```python
from build123d import *

# Parameters (mm, degrees)
SKETCH1_W           = 55.5
SKETCH1_H           = 25.6
SKETCH1_R           = 10
SKETCH1_W_2         = 5
SKETCH1_H_2         = 20
BOSS_EXTRUDE1_DEPTH = 21.5
BOSS_EXTRUDE2_START = 3
SKETCH1_2_W         = 5
SKETCH1_2_H         = 20
SKETCH1_2_R         = 10
BOSS_EXTRUDE2_DEPTH = 18.5


with BuildPart() as part:
    # Sketch1 → Boss-Extrude1 (new body)
    with BuildSketch(Plane.XY):
        Rectangle(SKETCH1_W, SKETCH1_H)
        with Locations((15.75, 0)):
            Circle(SKETCH1_R, mode=Mode.SUBTRACT)
        with Locations((-22.25, 0)):
            Rectangle(SKETCH1_W_2, SKETCH1_H_2, mode=Mode.SUBTRACT)
    extrude(amount=BOSS_EXTRUDE1_DEPTH)

    # Sketch1<2> → Boss-Extrude2 (add)
    with BuildSketch(Plane.XY.offset(BOSS_EXTRUDE2_START)):
        with Locations((-22.25, 0)):
            Rectangle(SKETCH1_2_W, SKETCH1_2_H)
        with Locations(Location((15.75, 0, 0), (0, 0, 180))):
            Circle(SKETCH1_2_R)
    extrude(amount=BOSS_EXTRUDE2_DEPTH)


solid = part.part
```
The listing builds one solid part. Answer for the finished solid, in the listing's coordinates (mm). A direction names the side the tool comes from. Round coordinates to 2 decimals unless told otherwise and drop trailing zeros. Loops run counter-clockwise (first coordinate to the right, second up) from the corner with the lowest first, then second, coordinate; pieces in that order, holes last. Notation, with made-up numbers: (14, -7.5) - (50, -7.5) arc R16 cw to (50, 7.5) - close; hole circle Ø3 at (53, 23.5). An arc over 180 degrees is marked (long way). Use one line per item in the form item = value. Start each with the question number.
1. The part is cut by section C-C on x = 7. Determine the outline of the cut face in (y, z), then the cut area to 3 significant figures.
2. The part is cut by section D-D on y = -6.75. Determine the outline of the cut face in (x, z), then the cut area to 3 significant figures.
3. Consider line 1 (Y direction, x = 15.75, z = 1.45); line 2 (X direction, y = 0.5, z = 1.5); line 3 (Z direction, x = 20, y = -3.5). Determine where each line is inside the solid, lowest interval first. Write a range as [from, to].
4. The part is cut by section A-A on x = 15.75. Determine the outline of the cut face in (y, z).
5. Given pin 1 Ø2 at (x, y) = (9, 4.5) entering from -Z, flat-ended and moving along its own axis, determine where the tip first touches the part or whether it passes through.
6. The part is cut by section B-B on y = 0. Determine the outline of the cut face in (x, z).
7. A tool of negligible diameter and unlimited length cuts with its end or side. For faces 1 (the face through (-7, 0, 0)), 2 (the face through (-22, 10, 1)), from which of +Z, -Z, +X, -X, +Y, -Y can it reach the whole face along a straight path? Write none if from no direction.
Geometry check:
q1.outline = (-12.8, 0) - (-4.84, 0) - (-4.84, 3) - (4.84, 3) - (4.84, 0) - (12.8, 0) - (12.8, 21.5) - (-12.8, 21.5) - close
q1.area = 521 mm^2
q2.outline = (-27.75, 0) - (-24.75, 0) - (-24.75, 3) - (-19.75, 3) - (-19.75, 0) - (8.37, 0) - (8.37, 3) - (23.13, 3) - (23.13, 0) - (27.75, 0) - (27.75, 21.5) - (-27.75, 21.5) - close
q2.area = 1,130 mm^2
q3.line_1 = [-12.8, -10], [10, 12.8]
q3.line_2 = [-27.75, -24.75], [-19.75, 5.76], [25.74, 27.75]
q3.line_3 = [3, 21.5]
q4.outline = (-12.8, 0) - (-10, 0) - (-10, 3) - (10, 3) - (10, 0) - (12.8, 0) - (12.8, 21.5) - (-12.8, 21.5) - close
q5.pin_1 = 3
q6.outline = (-27.75, 0) - (-24.75, 0) - (-24.75, 3) - (-19.75, 3) - (-19.75, 0) - (5.75, 0) - (5.75, 3) - (25.75, 3) - (25.75, 0) - (27.75, 0) - (27.75, 21.5) - (-27.75, 21.5) - close
q7.face_1 = -Z, +X, -X, +Y, -Y
q7.face_2 = -Z
